```python
from build123d import *

# Parameters (mm, degrees)
SKETCH_1_W          = 110
SKETCH_1_H          = 40
SKETCH_1_R          = 2.05
EXTRUDE_1_DEPTH     = 4
SKETCH_2_R          = 2.1
SKETCH_2_W          = 110
SKETCH_2_H          = 40
EXTRUDE_2_DEPTH     = 4
FILLET_3_R          = 10
FILLET_4_R          = 5
SKETCH_5_W          = 38.5
SKETCH_5_H          = 24
CUT_EXTRUDE_3_DEPTH = 10
CUT_EXTRUDE_4_DEPTH = 10
CUT_EXTRUDE_5_DEPTH = 10
FILLET_5_R          = 3
SKETCH_8_R          = 2.1
CUT_EXTRUDE_6_DEPTH = 10


with BuildPart() as part:
    # 草图1 → 凸台-拉伸1 (new body)
    with BuildSketch(Plane.XY):
        Rectangle(SKETCH_1_W, SKETCH_1_H)
        with Locations((-50, 14)):
            Circle(SKETCH_1_R, mode=Mode.SUBTRACT)
        with Locations((50, 14)):
            Circle(SKETCH_1_R, mode=Mode.SUBTRACT)
        with Locations((50, -14)):
            Circle(SKETCH_1_R, mode=Mode.SUBTRACT)
        with Locations((-50, -14)):
            Circle(SKETCH_1_R, mode=Mode.SUBTRACT)
    extrude(amount=EXTRUDE_1_DEPTH)

    # 草图2 → 凸台-拉伸2 (add)
    # profile 1 of 2: a face of its own
    with BuildSketch(Plane.XY.offset(4)):
        Polygon((-207.040642195, -115), (207.040642195, -115), (55, -60), (-55, -60), align=None)
        with Locations((150, -105)):
            Circle(SKETCH_2_R, mode=Mode.SUBTRACT)
        with Locations((75, -105)):
            Circle(SKETCH_2_R, mode=Mode.SUBTRACT)
        with Locations((0, -105)):
            Circle(SKETCH_2_R, mode=Mode.SUBTRACT)
        with Locations((-75, -105)):
            Circle(SKETCH_2_R, mode=Mode.SUBTRACT)
        with Locations((-150, -105)):
            Circle(SKETCH_2_R, mode=Mode.SUBTRACT)
    # profile 2 of 2: a face of its own
    with BuildSketch(Plane.XY.offset(4)):
        with Locations((0, -40)):
            Rectangle(SKETCH_2_W, SKETCH_2_H)
    extrude(amount=-EXTRUDE_2_DEPTH)

    # 圆角3
    fillet_3_edges = [part.edges().sort_by_distance(p)[0] for p in [
        (-207.040642195, -115, 2),
        (207.040642195, -115, 2),
    ]]
    fillet(fillet_3_edges, radius=FILLET_3_R)

    # 圆角4
    fillet_4_edges = [part.edges().sort_by_distance(p)[0] for p in [
        (55, -60, 2),
        (-55, -60, 2),
        (-55, 20, 2),
        (55, 20, 2),
    ]]
    fillet(fillet_4_edges, radius=FILLET_4_R)

    # 草图5 → 切除-拉伸3 (cut)
    with BuildSketch(Plane.XY.offset(4)):
        with Locations((-21.75, 0)):
            Rectangle(SKETCH_5_W, SKETCH_5_H)
        with Locations((21.75, 0)):
            Rectangle(SKETCH_5_W, SKETCH_5_H)
        Polygon((-3, -18), (-36.617445924, -18), (-3, -49.56760166), align=None)
        Polygon((-36.617445924, -18), (-41, -18), (-41, -22.115325169), (-4.382554076, -56.5), (-3, -55.201748001), (-3, -49.56760166), align=None)
        Polygon((-4.382554076, -56.5), (-41, -22.115325169), (-41, -90.884674831), align=None)
        Polygon((36.617445924, -18), (3, -18), (3, -49.56760166), align=None)
        Polygon((41, -18), (36.617445924, -18), (3, -49.56760166), (3, -55.201748001), (4.382554076, -56.5), (41, -22.115325169), align=None)
        Polygon((41, -22.115325169), (4.382554076, -56.5), (41, -90.884674831), align=None)
        Polygon((36.617445924, -95), (3, -63.43239834), (3, -95), align=None)
        Polygon((-3, -63.43239834), (-36.617445924, -95), (-3, -95), align=None)
    extrude(amount=-CUT_EXTRUDE_3_DEPTH, mode=Mode.SUBTRACT)

    # 草图6 → 切除-拉伸4 (cut)
    with BuildSketch(Plane.XY.offset(4)):
        with BuildLine():
            Line((-137.5, -100), (-87.5, -100))
            ThreePointArc((-87.5, -100), (-82.5, -105), (-87.5, -110))
            Line((-87.5, -110), (-137.5, -110))
            ThreePointArc((-137.5, -110), (-142.5, -105), (-137.5, -100))
        make_face()
        with BuildLine():
            Line((-62.5, -100), (-12.5, -100))
            ThreePointArc((-12.5, -100), (-7.5, -105), (-12.5, -110))
            Line((-12.5, -110), (-62.5, -110))
            ThreePointArc((-62.5, -110), (-67.5, -105), (-62.5, -100))
        make_face()
        with BuildLine():
            Line((12.5, -100), (62.5, -100))
            ThreePointArc((62.5, -100), (67.5, -105), (62.5, -110))
            Line((62.5, -110), (12.5, -110))
            ThreePointArc((12.5, -110), (7.5, -105), (12.5, -100))
        make_face()
        with BuildLine():
            Line((87.5, -100), (137.5, -100))
            ThreePointArc((137.5, -100), (142.5, -105), (137.5, -110))
            Line((137.5, -110), (87.5, -110))
            ThreePointArc((87.5, -110), (82.5, -105), (87.5, -100))
        make_face()
        Polygon((-53, -65.657022536), (-134.115002501, -95), (-53, -95), align=None)
        Polygon((134.115002501, -95), (53, -95), (53, -65.657022536), align=None)
    extrude(amount=-CUT_EXTRUDE_4_DEPTH, mode=Mode.SUBTRACT)

    # 草图7 → 切除-拉伸5 (cut)
    with BuildSketch(Plane.XY.offset(4)):
        Polygon((-3, -95), (3, -95), (3, -63.43239834), (0, -60.615325169), (-3, -63.43239834), align=None)
    extrude(amount=-CUT_EXTRUDE_5_DEPTH, mode=Mode.SUBTRACT)

    # 圆角5
    fillet_5_edges = [part.edges().sort_by_distance(p)[0] for p in [
        (3, -18, 2),
        (41, -18, 2),
        (41, -90.884674831, 2),
        (3, -55.201748001, 2),
        (36.617445924, -95, 2),
        (-3, -18, 2),
        (-3, -55.201748001, 2),
        (-41, -90.884674831, 2),
        (-41, -18, 2),
        (2.5, 12, 2),
        (41, 12, 2),
        (41, -12, 2),
        (2.5, -12, 2),
        (-36.617445924, -95, 2),
        (-2.5, 12, 2),
        (-2.5, -12, 2),
        (-41, -12, 2),
        (-41, 12, 2),
        (-53, -65.657022536, 2),
        (-53, -95, 2),
        (-134.115002501, -95, 2),
        (53, -65.657022536, 2),
        (134.115002501, -95, 2),
        (53, -95, 2),
        (0, -60.615325169, 2),
    ]]
    fillet(fillet_5_edges, radius=FILLET_5_R)

    # 草图8 → 切除-拉伸6 (cut)
    with BuildSketch(Plane.XY.offset(4)):
        with Locations((-47.5, -45)):
            Circle(SKETCH_8_R)
        with Locations((-47.5, -70)):
            Circle(SKETCH_8_R)
        with Locations((47.5, -45)):
            Circle(SKETCH_8_R)
        with Locations((47.5, -70)):
            Circle(SKETCH_8_R)
    extrude(amount=-CUT_EXTRUDE_6_DEPTH, mode=Mode.SUBTRACT)


solid = part.part
```
Source: CAD feature listing. Evaluate the final solid. Frame: model axes, mm. Coordinates: 2 decimals unless noted, no trailing zeros. Write each loop counter-clockwise with the first axis right and the second up, starting at its lowest first coordinate (ties: lowest second). Pieces come first, ordered by that corner, then holes. Notation, with made-up numbers: (10.25, 58.25) -> (65.25, 58.25) arc R31 cw to (65.25, 93.25) -> close; hole circle Ø2 at (45, 52). An arc over 180 degrees is marked (long way). Return JSON: item names as keys, results as strings. Group by question number.
1) Section query C-C, the plane z = 1.85. State how many separate pieces and enclosed holes the cut face has, plus the area to 3 significant figures.
2) Section query B-B, the plane x = -105.5. Return loops of the section in (y, z), plus the area to 3 significant figures.
3) Contact query for flat-ended pins moving along their axis: P1, Ø2, axis at x = -72.5, z = 2.5, coming from the +Y side; P2, Ø1.5, axis at x = 54, z = 3.5, coming from the +Y side; P3, Ø2, axis at x = 114, z = 1.5, coming from the +Y side. Output: stop coordinate, or through.
4) Mould query, pull axis Y, two halves, no side actions, for faces 1 (the face through (-13, -67, 4)), 2 (the face through (87.09, -77.99, 2.03)), 3 (the face through (-159.814, -106.919, 1.972)), 4 (the face through (-87.09, -77.99, 2.03)). Classes: +Y half, -Y half, draft (parallel to the pull), parting line (faces both ways), or undercut.
5) Section query A-A, the plane y = -35. Return loops of the section in (x, z), plus the area to 3 significant figures.
6) Ray query, line 1 along Y through (x, z) = (-50.5, 2.35); line 2 along X through (y, z) = (-35, 3); line 3 along X through (y, z) = (-4.5, 1.05). Return the intervals inside material, ascending.
From the geometry:
{
 "1": {"separate pieces": "1", "enclosed holes": "24", "area": "10,300 mm²"},
 "2": {"outline": "(-115, 0) -> (-110, 0) -> (-110, 4) -> (-115, 4) -> close; (-100, 0) -> (-95, 0) -> (-95, 4) -> (-100, 4) -> close; (-84.65, 0) -> (-78.27, 0) -> (-78.27, 4) -> (-84.65, 4) -> close", "area": "65.5 mm²"},
 "3": {"P1": "y = -65.97", "P2": "y = 18.8", "P3": "y = -80.98"},
 "4": {"face 1": "draft", "face 2": "undercut", "face 3": "parting line", "face 4": "undercut"},
 "5": {"outline": "(-55, 0) -> (-41, 0) -> (-41, 4) -> (-55, 4) -> close; (-3, 0) -> (3, 0) -> (3, 4) -> (-3, 4) -> close; (41, 0) -> (55, 0) -> (55, 4) -> (41, 4) -> close", "area": "136 mm²"},
 "6": {"line 1": "-115 to -110, -100 to -15.99, -12.01 to 12.01, 15.99 to 19.97", "line 2": "-55 to -41, -3 to 3, 41 to 55", "line 3": "-55 to -41, -2.5 to 2.5, 41 to 55"}
}
